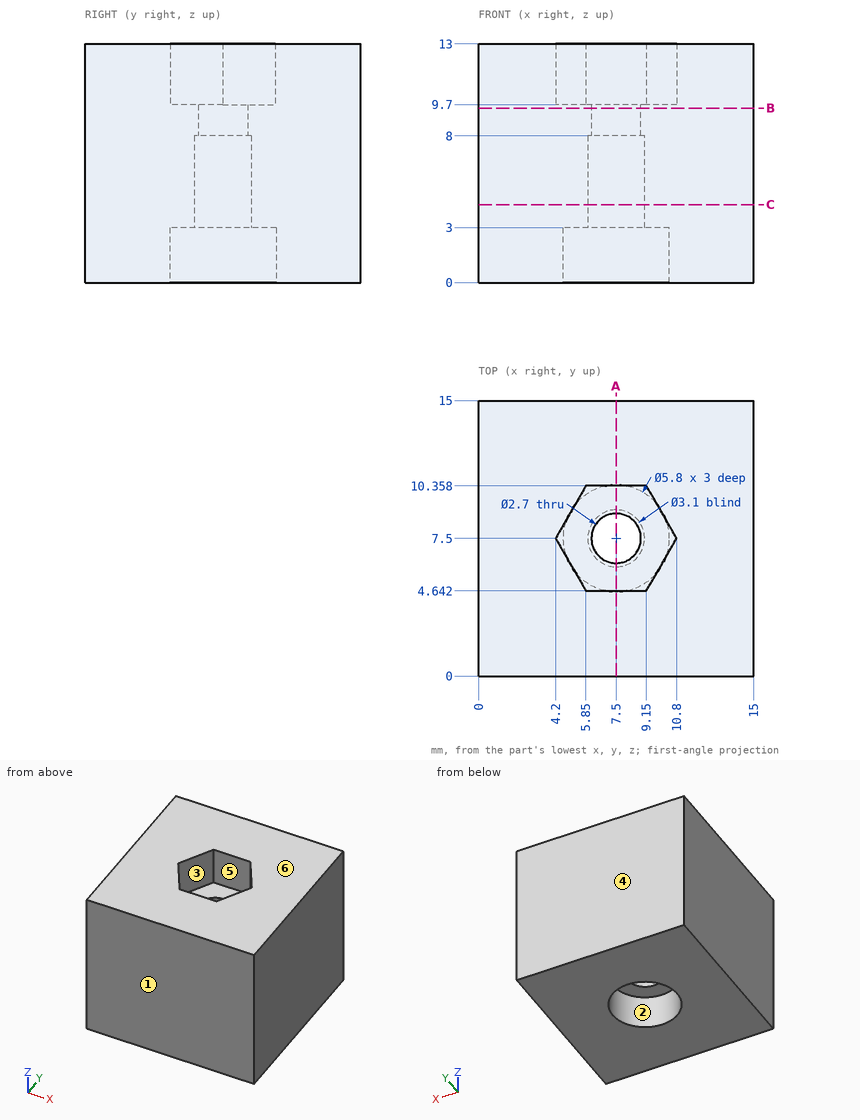
Here's the drawing with two shaded views (mm, measured from the low corner). I have some questions. A direction names the side the tool comes from. Round coordinates to 2 decimals unless told otherwise and drop trailing zeros. Order: outer loops, then holes, each group sorted by start corner. A loop starts at its lowest first (then second) coordinate and runs counter-clockwise, first axis right, second up. Notation, with made-up numbers: (-8, 75) -> (38, 75) arc R30 ccw to (38, 104) -> close; hole circle Ø6 at (-1.75, 4). An arc over 180 degrees is marked (long way). Return JSON: item names as keys, results as strings.
Q1. I need wall thicknesses on line 1 along Y through (x, z) = (7.5, 8.95); line 2 along Y through (x, z) = (9, 12.75); line 3 along X through (y, z) = (6.75, 2.75). Which ranges of each line are inside material? Lowest first, please. Write a range as from..to.
Filled sheet:
{"line 1": "y = 0..6.15, 8.85..15", "line 2": "y = 0..4.64, 10.36..15", "line 3": "x = 0..4.7, 10.3..15"}
Q2. If we section it at B-B on z = 9.5: List the corners of the cut face in (x, y) for me, plus the area to 3 significant figures.
Filled sheet:
{"outline": "(0, 0) -> (15, 0) -> (15, 15) -> (0, 15) -> close; hole circle Ø2.7 at (7.5, 7.5)", "area": "219 mm^2"}
Q3. For pin 1 Ø3.5 at (x, y) = (7.5, 7.5) entering from -Z, with a flat end and sliding along its axis, tell me the tip position at first contact or that it passes through.
Filled sheet:
{"pin 1": "stops at z = 3"}
Q4. If we mould it in two halves opening along Y, with no side actions, what happens to the marked faces 4, 5 and 6? For each: released by +Y, released by -Y, zero draft, split by the parting line, or undercut.
Filled sheet:
{"face 4": "released by +Y", "face 5": "undercut", "face 6": "zero draft"}
Q5. If we section it at C-C on z = 4.25: List the corners of the cut face in (x, y) for me, plus the area to 3 significant figures.
Filled sheet:
{"outline": "(0, 0) -> (15, 0) -> (15, 15) -> (0, 15) -> close; hole circle Ø3.1 at (7.5, 7.5)", "area": "217 mm^2"}
Q6. Which directions (+Z, -Z, +X, -X, +Y, -Y) give clear straight access to the entire face, cutting with the end or side of a thin tool? Please do the marked faces 1, 2 and 3.
Filled sheet:
{"face 1": "+Z, -Z, +X, -X, -Y", "face 2": "-Z", "face 3": "+Z"}
Q7. If we section it at A-A on x = 7.5: List the corners of the cut face in (y, z) for me.
Filled sheet:
{"outline": "(0, 0) -> (4.6, 0) -> (4.6, 3) -> (5.95, 3) -> (5.95, 8) -> (6.15, 8) -> (6.15, 9.7) -> (4.64, 9.7) -> (4.64, 13) -> (0, 13) -> close; (8.85, 8) -> (9.05, 8) -> (9.05, 3) -> (10.4, 3) -> (10.4, 0) -> (15, 0) -> (15, 13) -> (10.36, 13) -> (10.36, 9.7) -> (8.85, 9.7) -> close"}
